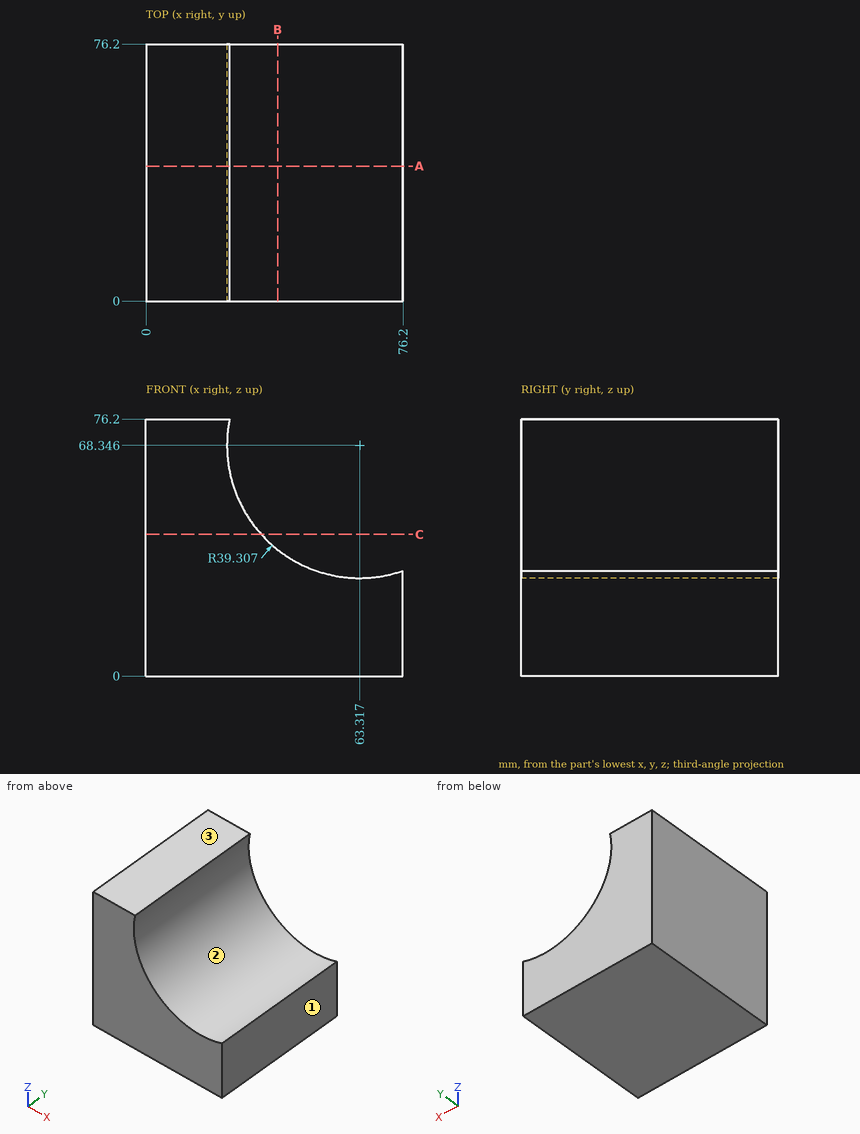
Geometry: see drawing. Coordinates: mm, zero at the bounding-box minimum. Round coordinates to 2 decimals unless told otherwise and drop trailing zeros. Write each loop counter-clockwise with the first axis right and the second up, starting at its lowest first coordinate (ties: lowest second). Pieces come first, ordered by that corner, then holes. Notation, with made-up numbers: M 52.5,31.25 L 87.5,31.25 A25 cw 87.5,59.25 Z; hole C 53.5,-22.5 d3. An arc over 180 degrees is marked long. Answer in a Markdown table with one row per item. Add a question column.
(1) Draft query along Z for the marked faces 1, 2 and 3. Return one class per face: pulls with the +Z half, pulls with the -Z half, needs draft (parallel to the pull), parting line crosses it, or undercut.
(2) Cut plane C-C, the plane z = 42. Return the cut outline in (x, y), then the cut area to 3 significant figures.
(3) Cut plane A-A, the plane y = 40. Return the cut outline in (x, z), then the cut area to 3 significant figures.
(4) Ray query, L1, parallel to Z at x = 44, y = 23 (1 decimal); L2, parallel to Z at x = 37, y = 12.5; L3, parallel to X at y = 8, z = 46. Return the intervals inside material, ascending.
(5) Cut plane B-B, the plane x = 39. Return the cut outline in (y, z) (1 decimal).
(6) Contact query for flat-ended pins moving along their axis: pin 1 (4 mm diameter, centred on x = 29, y = 52.5, fed in from -Z); pin 2 (3 mm diameter, centred on y = 56, z = 62, fed in from +X); pin 3 (2 mm diameter, centred on x = 42.5, y = 41.5, fed in from +Z); pin 4 (1 mm diameter, centred on x = 41.5, y = 18, fed in from +Z). Output: stop coordinate, or through.
Established:
| question | item | result |
|---|---|---|
| 1 | face 1 | needs draft |
| 1 | face 2 | undercut |
| 1 | face 3 | pulls with the +Z half |
| 2 | outline | M 0,0 L 34.15,0 L 34.15,76.2 L 0,76.2 Z |
| 2 | area | 2,600 mm² |
| 3 | outline | M 0,0 L 76.2,0 L 76.2,31.21 A39.31 cw 24.8,76.2 L 0,76.2 Z |
| 3 | area | 3,690 mm² |
| 4 | L1 | 0 to 34.1 |
| 4 | L2 | 0 to 39.15 |
| 4 | L3 | 0 to 30.98 |
| 5 | outline | M 0,0 L 76.2,0 L 76.2,37.5 L 0,37.5 Z |
| 6 | pin 1 | z = 0 |
| 6 | pin 2 | x = 24.8 |
| 6 | pin 3 | z = 35.65 |
| 6 | pin 4 | z = 35.99 |
